Work out the finished part from the listing and answer in its coordinate system (mm). Give positions to 0.01 mm unless a question says otherwise; leave off trailing zeros. Order: outer loops, then holes, each group sorted by start corner. A loop starts at its lowest first (then second) coordinate and runs counter-clockwise, first axis right, second up. Notation, with made-up numbers: M 38,-6.75 L 71,-6.75 A18 ccw 71,11.25 Z; hole C 2,-11.75 d10. An arc over 180 degrees is marked long. One line per item, written item: value.
from build123d import *

# Parameters (mm, degrees)
SKETCH_1_R          = 2.1
SKETCH_1_R_2        = 6
EXTRUDE_1_DEPTH     = 24
FILLET_1_R          = 2.5
CUT_EXTRUDE_START   = -24
SKETCH_3_R          = 1.6
SKETCH_3_R_2        = 1.5
SKETCH_3_R_3        = 2.1
CUT_EXTRUDE_2_DEPTH = 24


with BuildPart() as part:
    # 草图1 → 凸台-拉伸1 (new body)
    # profile 1 of 3: a face of its own
    with BuildSketch(Plane.XY):
        with BuildLine():
            Line((68.135486627, 53), (-0.671642545, 53))
            ThreePointArc((-0.671642545, 53), (15.918389352, 49.295479077), (29.356722765, 38.885684233))
            Line((29.356722765, 38.885684233), (68.135486627, 53))
        make_face()
    # profile 2 of 3: a face of its own
    with BuildSketch(Plane.XY):
        with BuildLine():
            ThreePointArc((29.356722765, 38.885684233), (15.918389352, 49.295479077), (-0.671642545, 53))
            ThreePointArc((-0.671642545, 53), (-20.639649059, 47.500428563), (-34.976092597, 32.552754602))
            ThreePointArc((-34.976092597, 32.552754602), (-28.226351446, 35.515083761), (-23.69848481, 29.69848481))
            ThreePointArc((-23.69848481, 29.69848481), (-24.155207625, 27.402384191), (-25.45584416, 25.455844085))
            ThreePointArc((-25.45584416, 25.455844085), (-6.992802508, 35.314313148), (13.833943007, 33.235854448))
            Line((13.833943007, 33.235854448), (29.356722765, 38.885684233))
        make_face()
        with Locations((0, 42)):
            Circle(SKETCH_1_R, mode=Mode.SUBTRACT)
    # profile 3 of 3: a face of its own
    with BuildSketch(Plane.XY):
        with Locations((-29.69848481, 29.69848481)):
            Circle(SKETCH_1_R_2)
        with Locations((-29.69848481, 29.69848481)):
            Circle(SKETCH_1_R, mode=Mode.SUBTRACT)
    extrude(amount=EXTRUDE_1_DEPTH)

    # 圆角1
    fillet_1_edges = [part.edges().sort_by_distance(p)[0] for p in [
        (68.135486627, 53, 12),
    ]]
    fillet(fillet_1_edges, radius=FILLET_1_R)

    # 草图3 → 切除-拉伸2 (cut)
    with BuildSketch(Plane.XY.offset(24).offset(CUT_EXTRUDE_START)):
        with Locations((11, 49)):
            Circle(SKETCH_3_R)
        with Locations((31, 49)):
            Circle(SKETCH_3_R_2)
        with Locations((0, 42)):
            Circle(SKETCH_3_R_3)
    extrude(amount=CUT_EXTRUDE_2_DEPTH, mode=Mode.SUBTRACT)


solid = part.part
(1) Section D-D, the plane x = 28.5 is taken. Give the vertices of the cut face in (y, z).
Findings:
outline: M 38.57,0 L 53,0 L 53,24 L 38.57,24 Z
(2) Section C-C, the plane z = 18.25 is taken. Give the vertices of the cut face in (x, y).
Findings:
outline: M -34.98,32.55 A6 ccw -25.46,25.46 A36 cw 13.83,33.24 L 54.81,48.15 A2.5 ccw 53.96,53 L -0.67,53 A39 ccw Z; hole C -29.7,29.7 d4.2; hole C 0,42 d4.2; hole C 11,49 d3.2; hole C 31,49 d3
(3) Determine the mould class of faces 1 (the cylindrical face through (56.41, 50.98, 12.17)), 2 (the cylindrical face through (9.4, 49.07, 11.83)), 3 (the cylindrical face through (-7.284, 35.255, 11.832)), 4 (the cylindrical face through (30.675, 47.536, 11.832)) for opening direction Y: pulls with the +Y half, pulls with the -Y half, needs draft (parallel to the pull), parting line crosses it, or undercut.
Findings:
face 1: parting line crosses it
face 2: undercut
face 3: pulls with the -Y half
face 4: undercut
(4) Given P1, Ø1, axis at x = -25.5, z = 14, coming from the +Y side; P2, Ø1.9, axis at x = 11, y = 49, coming from the +Z side; P3, Ø8, axis at x = -8, z = 7.5, coming from the +Y side; P4, Ø1.5, axis at y = 36, z = 3, coming from the -X side, each flat-ended and moving along its own axis, determine where each tip first touches the part or whether it passes through.
Findings:
P1: stops at y = 44.48
P2: passes through
P3: stops at y = 52.86
P4: stops at x = -33.37
(5) Section A-A, the plane y = 34.75 is taken. Give the vertices of the cut face in (x, z).
Findings:
outline: M -33.69,0 L -9.4,0 L -9.4,24 L -33.69,24 Z; M 9.4,0 L 17.99,0 L 17.99,24 L 9.4,24 Z
(6) Find the intervals of material crossed by probe 1 along Y at (x, z) = (0, 16.75); probe 2 along Y at (x, z) = (11, 6.75); probe 3 along Y at (x, z) = (6, 10.5), in increasing order. Write a range as from..to.
Findings:
probe 1: y = 36..39.9, 44.1..53
probe 2: y = 34.28..47.4, 50.6..53
probe 3: y = 35.5..53
(7) Section B-B, the plane x = 11.5 is taken. Give the vertices of the cut face in (y, z), then the cut area to 3 significant figures.
Findings:
outline: M 34.11,0 L 47.48,0 L 47.48,24 L 34.11,24 Z; M 50.52,0 L 53,0 L 53,24 L 50.52,24 Z
area: 380 mm^2
